Design review of the part built by this model. Coordinates are the model's own, in mm. Coordinates: 2 decimals unless noted, no trailing zeros. Loops run counter-clockwise (first coordinate to the right, second up) from the corner with the lowest first, then second, coordinate; pieces in that order, holes last. Notation, with made-up numbers: (71.5, -11) - (76.5, -11) arc R33 ccw to (76.5, 18) - close; hole circle Ø5 at (88, -4.5). An arc over 180 degrees is marked (long way). Answer in a Markdown table with one row per item. Add a question column.
(1) To check wall thickness, follow L1, parallel to Y at x = 2.5, z = 1.1; L2, parallel to Y at x = -9.5, z = 1.4; L3, parallel to X at y = -0.75, z = 2.35. State the ranges of each line that lie inside material, in increasing order. Write a range as [from, to].
(2) The part is to be moulded in two halves that separate along X. For faces 1 (the face through (-14.985, 0.66, 1.479)), 2 (the face through (-0.417, 0.759, 1.479)), 3 (the face through (0, 0, 0)), say which applies: released by +X, released by -X, zero draft, split by the parting line, or undercut.
(3) We need section D-D, the plane x = -6. Write out the cut boundary in (y, z), plus the area to 3 significant figures.
(4) We need section C-C, the plane y = -7.5. Write out the cut boundary in (x, z).
(5) We need section B-B, the plane x = 9.5. Write out the cut boundary in (y, z), plus the area to 3 significant figures.
(6) We need section A-A, the plane z = 1.85. Write out the cut boundary in (x, y).
(7) Clearance check with a flat-ended pin moving along its axis: pin 1 (1.6 mm diameter, centred on x = -1.32, y = 0.72, fed in from +Z). State where the tip first meets the part, or that it passes through.
from build123d import *

# Parameters (mm, degrees)
SKETCH1_R           = 15
BOSS_EXTRUDE1_DEPTH = 3
SKETCH2_R           = 0.9
CUT_EXTRUDE1_DEPTH  = 3


with BuildPart() as part:
    # Sketch1 → Boss-Extrude1 (new body)
    with BuildSketch(Plane.XY):
        Circle(SKETCH1_R)
    extrude(amount=BOSS_EXTRUDE1_DEPTH)

    # Sketch2 → Cut-Extrude1 (cut)
    with BuildSketch(Plane(origin=(0, 0, 0), x_dir=(-1, 0, 0), z_dir=(0, 0, -1))):
        with Locations((-1.31599788, -0.719826076)):
            Circle(SKETCH2_R)
        with Locations((1.31599788, 0.719826076)):
            Circle(SKETCH2_R)
        with Locations((-3.011222811, -9.535855346)):
            Circle(SKETCH2_R)
        with Locations((-9.535855346, 3.011222811)):
            Circle(SKETCH2_R)
        with Locations((3.011222811, 9.535855346)):
            Circle(SKETCH2_R)
        with Locations((9.535855346, -3.011222811)):
            Circle(SKETCH2_R)
    extrude(amount=-CUT_EXTRUDE1_DEPTH, mode=Mode.SUBTRACT)


solid = part.part
Responses:
| question | item | result |
|---|---|---|
| 1 | L1 | y = [-14.79, -10.28], [-8.8, 14.79] |
| 1 | L2 | y = [-11.61, -3.91], [-2.11, 11.61] |
| 1 | L3 | x = [-14.98, 0.42], [2.22, 14.98] |
| 2 | face 1 | split by the parting line |
| 2 | face 2 | undercut |
| 2 | face 3 | zero draft |
| 3 | outline | (-13.75, 0) - (13.75, 0) - (13.75, 3) - (-13.75, 3) - close |
| 3 | area | 82.5 mm2 |
| 4 | outline | (-12.99, 0) - (12.99, 0) - (12.99, 3) - (-12.99, 3) - close |
| 5 | outline | (-11.61, 0) - (2.11, 0) - (2.11, 3) - (-11.61, 3) - close; (3.91, 0) - (11.61, 0) - (11.61, 3) - (3.91, 3) - close |
| 5 | area | 64.3 mm2 |
| 6 | outline | circle Ø30 at (0, 0); hole circle Ø1.8 at (-9.54, -3.01); hole circle Ø1.8 at (-3.01, 9.54); hole circle Ø1.8 at (-1.32, 0.72); hole circle Ø1.8 at (1.32, -0.72); hole circle Ø1.8 at (3.01, -9.54); hole circle Ø1.8 at (9.54, 3.01) |
| 7 | pin 1 | passes through |
